CAD build for the part. Positions are in the model's coordinates, mm. A direction names the side the tool comes from. Give positions to 0.01 mm unless a question says otherwise; leave off trailing zeros. Order: outer loops, then holes, each group sorted by start corner. A loop starts at its lowest first (then second) coordinate and runs counter-clockwise, first axis right, second up.
Item 1: Flat gauge pins, fed straight in: P1, Ø4, axis at x = -40, z = 85, coming from the +Y side; P2, Ø1.5, axis at x = -28.5, y = 1, coming from the -Z side; P3, Ø1, axis at x = 11, y = 2, coming from the +Z side; P4, Ø1.5, axis at y = 2.5, z = -9, coming from the +X side. Where does each tip first touch, or does it go through?
Item 2: Which spindle directions (+Z, -Z, +X, -X, +Y, -Y) get a long thin tool onto all of the face, cutting with end or side? Do faces 1 (the cylindrical face through (9, 1, 13)), 2 (the flat face through (1, 3, 21)). Say none if no direction does.
Item 3: Band-saw the part on A-A on x = 65. Give the cut face in (y, z).
Item 4: Band-saw the part on D-D on x = -76.5. Give the cut face in (y, z), plus the area to 3 significant figures.
Item 5: Wall check: L1, parallel to Z at x = -44.5, y = 1.05; L2, parallel to X at y = 1.1, z = 85; L3, parallel to Z at x = 81, y = 2.75. Give the ranges that are in metal, low to high.
Item 6: Band-saw the part on B-B on y = 0.6. Count the separate pieces of the cut face and the enclosed holes in it, plus the area to 3 significant figures.
Item 7: Band-saw the part on C-C on x = -32. Give the cut face in (y, z).
Item 8: Two-plate mould, pull along Z, no slides. Class faces 3 (the cylindrical face through (8, 1, -14)), 4 (the cylindrical face through (30.04, 1.48, 95.38)), 5 (the flat face through (1, 0, 21)), 6 (the cylindrical face through (-43, 1, 14)): released by +Z, released by -Z, zero draft, split by the parting line, or undercut.
```python
from build123d import *

# Parameters (mm, degrees)
CROQUIS1_R              = 100
CROQUIS1_R_2            = 1.65
CROQUIS1_R_3            = 10.25
CROQUIS1_R_4            = 1.1
CROQUIS1_W              = 19.5
CROQUIS1_H              = 12.5
SALIENTE_EXTRUIR1_DEPTH = 3


with BuildPart() as part:
    # Croquis1 → Saliente-Extruir1 (new body)
    with BuildSketch(Plane(origin=(0, 0, 0), x_dir=(1, 0, 0), z_dir=(0, 1, 0))):
        with Locations(Location((0, 0, 0), (0, 0, 270))):
            Circle(CROQUIS1_R)
        with Locations(Location((55, 75, 0), (0, 0, 270))):
            Circle(CROQUIS1_R_2, mode=Mode.SUBTRACT)
        with Locations(Location((40, -85, 0), (0, 0, 270))):
            Circle(CROQUIS1_R_2, mode=Mode.SUBTRACT)
        with Locations(Location((40, 85, 0), (0, 0, 90))):
            Circle(CROQUIS1_R_2, mode=Mode.SUBTRACT)
        with Locations(Location((-60.20239259, 39.027979594, 0), (0, 0, 270))):
            Circle(CROQUIS1_R_2, mode=Mode.SUBTRACT)
        with Locations(Location((-40, -85, 0), (0, 0, 90))):
            Circle(CROQUIS1_R_2, mode=Mode.SUBTRACT)
        with Locations(Location((-55, -75, 0), (0, 0, 270))):
            Circle(CROQUIS1_R_2, mode=Mode.SUBTRACT)
        with Locations(Location((-55, 75, 0), (0, 0, 90))):
            Circle(CROQUIS1_R_2, mode=Mode.SUBTRACT)
        with Locations(Location((-40, 85, 0), (0, 0, 270))):
            Circle(CROQUIS1_R_2, mode=Mode.SUBTRACT)
        with Locations(Location((-60.20239259, 9.027979594, 0), (0, 0, 270))):
            Circle(CROQUIS1_R_2, mode=Mode.SUBTRACT)
        with Locations(Location((72.25, 40, 0), (0, 0, 270))):
            Circle(CROQUIS1_R_3, mode=Mode.SUBTRACT)
        with Locations(Location((-43.20239259, 36.8, 0), (0, 0, 270))):
            Circle(CROQUIS1_R_2, mode=Mode.SUBTRACT)
        with Locations(Location((8.29760741, 70, 0), (0, 0, 270))):
            Circle(CROQUIS1_R_2, mode=Mode.SUBTRACT)
        with Locations(Location((21, -57, 0), (0, 0, 90))):
            Circle(CROQUIS1_R_2, mode=Mode.SUBTRACT)
        with Locations(Location((-27, -24, 0), (0, 0, 90))):
            Circle(CROQUIS1_R_2, mode=Mode.SUBTRACT)
        with Locations(Location((55, -75, 0), (0, 0, 90))):
            Circle(CROQUIS1_R_2, mode=Mode.SUBTRACT)
        with Locations(Location((-22.18239259, 88.81, 0), (0, 0, 270))):
            Circle(CROQUIS1_R_4, mode=Mode.SUBTRACT)
        with Locations(Location((-17.10239259, 81.19, 0), (0, 0, 270))):
            Circle(CROQUIS1_R_4, mode=Mode.SUBTRACT)
        with BuildLine():
            Line((-40, 15), (5, 15))
            ThreePointArc((5, 15), (8.535533906, 13.535533906), (10, 10))
            Line((10, 10), (10, -10))
            ThreePointArc((10, -10), (8.535533906, -13.535533906), (5, -15))
            Line((5, -15), (-40, -15))
            ThreePointArc((-40, -15), (-43.535533906, -13.535533906), (-45, -10))
            Line((-45, -10), (-45, 10))
            ThreePointArc((-45, 10), (-43.535533906, 13.535533906), (-40, 15))
        make_face(mode=Mode.SUBTRACT)
        with Locations((72.25, -0.158534098)):
            Rectangle(CROQUIS1_W, CROQUIS1_H, mode=Mode.SUBTRACT)
    extrude(amount=SALIENTE_EXTRUIR1_DEPTH)


solid = part.part
```
The answers:
1. P1: stops at y = 3
1. P2: stops at z = -96.07
1. P3: stops at z = 99.45
1. P4: stops at x = 99.66
2. face 1: +Y, -Y
2. face 2: +Z, -Z, +X, -X, +Y
3. outline: (0, -75.99) - (3, -75.99) - (3, -47.25) - (0, -47.25) - close; (0, -32.75) - (3, -32.75) - (3, -6.09) - (0, -6.09) - close; (0, 6.41) - (3, 6.41) - (3, 75.99) - (0, 75.99) - close
4. outline: (0, -64.4) - (3, -64.4) - (3, 64.4) - (0, 64.4) - close
4. area: 386 mm2
5. L1: z = -89.55 to -37.82, -35.78 to -12.18, 12.18 to 89.55
5. L2: x = -52.68 to -41.65, -38.35 to 38.35, 41.65 to 52.68
5. L3: z = -58.64 to -45.34, -34.66 to -6.09, 6.41 to 58.64
6. separate pieces: 1
6. enclosed holes: 19
6. area: 29,100 mm2
7. outline: (0, -94.74) - (3, -94.74) - (3, -15) - (0, -15) - close; (0, 15) - (3, 15) - (3, 94.74) - (0, 94.74) - close
8. face 3: undercut
8. face 4: split by the parting line
8. face 5: zero draft
8. face 6: undercut
